CAD build for the part. Positions are in the model's coordinates, mm. A direction names the side the tool comes from. Round coordinates to 2 decimals unless told otherwise and drop trailing zeros. Order: outer loops, then holes, each group sorted by start corner. A loop starts at its lowest first (then second) coordinate and runs counter-clockwise, first axis right, second up.
```python
from build123d import *

# Parameters (mm, degrees)
SKETCH2_W               = 210
SKETCH2_H               = 160
BOSS_EXTRUDE1_DEPTH     = 10
SKETCH3_R               = 19.2
SKETCH3_W               = 41
SKETCH3_H               = 45
CUT_EXTRUDE2_DEPTH      = 15
CUT_EXTRUDE2_DEPTH_BACK = 22


with BuildPart() as part:
    # Sketch2 → Boss-Extrude1 (new body)
    with BuildSketch(Plane(origin=(0, 0, 0), x_dir=(1, 0, 0), z_dir=(0, 1, 0))):
        with Locations((5, 5)):
            Rectangle(SKETCH2_W, SKETCH2_H)
    extrude(amount=BOSS_EXTRUDE1_DEPTH)

    # Sketch3 → Cut-Extrude2 (cut, two sides)
    with BuildSketch(Plane(origin=(0, 0, 0), x_dir=(1, 0, 0), z_dir=(0, 1, 0))) as cut_extrude2_sk:
        with Locations((41.585, 0)):
            Circle(SKETCH3_R)
        with Locations((-45.952707493, 0)):
            Rectangle(SKETCH3_W, SKETCH3_H)
    extrude(amount=CUT_EXTRUDE2_DEPTH, mode=Mode.SUBTRACT)
    extrude(cut_extrude2_sk.sketch, amount=-CUT_EXTRUDE2_DEPTH_BACK, mode=Mode.SUBTRACT)


solid = part.part
```
1. Cut at A-A, the plane z = 0. Write the cut outline in (x, y) (3 decimals), and give its area (3 significant figures).
2. Cut at C-C, the plane y = 7.5. Write the cut outline in (x, z) (3 decimals).
3. Mould opens along X. For faces 1 (the face through (110, 5, -4)), 2 (the face through (4, 5, -85)), 3 (the face through (-46, 5, -22.5)), 4 (the face through (-25.453, 5, 0)) say: released by +X, released by -X, zero draft, split by the parting line, or undercut.
4. Cut at B-B, the plane x = -40. Write the cut outline in (y, z).
5. Pin check, flat tip, straight feed: P1, Ø6, axis at x = -59, z = 41.5, coming from the -Y side. Stop position of the tip, or through.
6. Drill centre lines: line 1 (X direction, y = 7.25, z = 0) (3 decimals); line 2 (Z direction, x = 41, y = 4.25); line 3 (Z direction, x = -29.5, y = 6.5). Where is each one in solid material? Low to high.
7. Tool access for faces 5 (the face through (4, 10, -6)), 6 (the face through (-46, 5, 22.5)): list every direction of +Z, -Z, +X, -X, +Y, -Y with a clear straight run to the whole face (end or side of a thin tool).
Outcome:
1. outline: (-100, 0) - (-66.453, 0) - (-66.453, 10) - (-100, 10) - close; (-25.453, 0) - (22.385, 0) - (22.385, 10) - (-25.453, 10) - close; (60.785, 0) - (110, 0) - (110, 10) - (60.785, 10) - close
1. area: 1,310 mm2
2. outline: (-100, -85) - (110, -85) - (110, 75) - (-100, 75) - close; hole (-66.453, -22.5) - (-25.453, -22.5) - (-25.453, 22.5) - (-66.453, 22.5) - close; hole circle Ø38.4 at (41.585, 0)
3. face 1: released by +X
3. face 2: zero draft
3. face 3: undercut
3. face 4: undercut
4. outline: (0, -85) - (10, -85) - (10, -22.5) - (0, -22.5) - close; (0, 22.5) - (10, 22.5) - (10, 75) - (0, 75) - close
5. P1: stops at y = 0
6. line 1: x = -100 to -66.453, -25.453 to 22.385, 60.785 to 110
6. line 2: z = -85 to -19.19, 19.19 to 75
6. line 3: z = -85 to -22.5, 22.5 to 75
7. face 5: +Z, -Z, +X, -X, +Y
7. face 6: +Y, -Y
